For this review, take the finished solid that the model builds, in its own axes (mm). A direction names the side the tool comes from. Give positions to 0.01 mm unless a question says otherwise; leave off trailing zeros. Loops run counter-clockwise (first coordinate to the right, second up) from the corner with the lowest first, then second, coordinate; pieces in that order, holes last. Notation, with made-up numbers: (-35, 85.25) - (-5, 85.25) arc R16 ccw to (-5, 113.25) - close; hole circle Ø9 at (-12, 20). An arc over 180 degrees is marked (long way). Use CSV: the item, a comma, the result in double quotes. Start each with the question number.
1. Take a section at D-D on y = 1. Give the boundary of the cut face in (x, z), plus the area to 3 significant figures.
2. Take a section at A-A on x = 0. Give the boundary of the cut face in (y, z).
3. For faces 1 (the cylindrical face through (-26.2, 22.8, 10)), 2 (the cylindrical face through (28.549, 24.055, 1.452)), 3 (the flat face through (-11, 19.55, 0)), list the 3-axis set-ups (+Z, -Z, +X, -X, +Y, -Y) from which the entire face can be reached by the end or side of a thin tool; tool diameter is ignored.
4. Take a section at B-B on y = 9.25. Give the boundary of the cut face in (x, z).
5. For pin 1 (9.5 mm diameter, centred on y = 13, z = 0, fed in from -X); pin 2 (12 mm diameter, centred on y = 9, z = 2, fed in from +X); pin 3 (5 mm diameter, centred on y = 11, z = 2, fed in from +X); pin 4 (3 mm diameter, centred on x = 0, z = 0, fed in from -Y), all flat-tipped, find the tip position at first contact; note any pin that passes through.
6. Wall thickness on line 1 (Y direction, x = -28, z = 0); line 2 (Z direction, x = -21.5, y = 13.5); line 3 (X direction, y = 7.75, z = 1): over which ranges is each line inside the solid? List them lowest first.
7. Mouldability with a two-part tool opening along Z and no side actions: class faces 4 (the flat face through (-32, 2, -6)), 5 (the cylindrical face through (23.03, 5.19, 1.73)), 6 (the cylindrical face through (17, 27, 0)), 7 (the cylindrical face through (-1.2, 2.2, -7.9)) as pulls with the +Z half, pulls with the -Z half, needs draft (parallel to the pull), parting line crosses it, or undercut.
```python
from build123d import *

# Parameters (mm, degrees)
SKETCH1_R                       = 26
SKETCH1_R_2                     = 21.249999999999996
BOSS_EXTRUDE1_DEPTH             = 9
BOSS_EXTRUDE2_START             = 2
SKETCH2_R                       = 26.000000000000007
SKETCH2_R_2                     = 21.249999999999996
BOSS_EXTRUDE2_DEPTH             = 2
BOSS_EXTRUDE3_REACH             = 40.38
BOSS_EXTRUDE3_DIRECTION_2_DEPTH = 18
SKETCH4_R                       = 11.15
CUT_EXTRUDE1_DEPTH              = 7
CUT_EXTRUDE2_START              = -7
SKETCH5_R                       = 11.15
CUT_EXTRUDE2_DEPTH              = 7
FILLET2_R                       = 14
FILLET4_R                       = 1
SKETCH8_W                       = 43.8178046004133
SKETCH8_H                       = 27.999999999999993
BOSS_EXTRUDE4_DEPTH             = 11
SKETCH9_W                       = 43.8178046004133
SKETCH9_H                       = 11.999999999999998
CUT_EXTRUDE4_DEPTH              = 45.988887516807985
BOSS_EXTRUDE5_DEPTH             = 42.5
SKETCH6_R                       = 8
CUT_EXTRUDE3_DEPTH              = 65.6065012208524
BOSS_EXTRUDE6_START             = -4
BOSS_EXTRUDE6_DEPTH             = 42
SKETCH11_R                      = 2
CUT_EXTRUDE5_DEPTH              = 46.39823785126468
CUT_EXTRUDE6_DEPTH              = 51.36864114704705


with BuildPart() as part:
    # Sketch1 → Boss-Extrude1 (new body)
    with BuildSketch(Plane(origin=(0, 0, 0), x_dir=(1, 0, 0), z_dir=(0, 1, 0))):
        with Locations(Location((0, 0, 0), (0, 0, 270))):
            Circle(SKETCH1_R)
        with Locations(Location((0, 0, 0), (0, 0, 270))):
            Circle(SKETCH1_R_2, mode=Mode.SUBTRACT)
    extrude(amount=BOSS_EXTRUDE1_DEPTH)

    # Sketch2 → Boss-Extrude2 (add)
    with BuildSketch(Plane.XZ.offset(BOSS_EXTRUDE2_START)):
        with Locations(Location((0, 0, 0), (0, 0, 270))):
            Circle(SKETCH2_R)
        with Locations(Location((0, 0, 0), (0, 0, 270))):
            Circle(SKETCH2_R_2, mode=Mode.SUBTRACT)
    extrude(amount=-BOSS_EXTRUDE2_DEPTH)

    # Boss-Extrude3: up to this face of the body (flat: up to its plane)
    boss_extrude3_end = Plane(part.part.faces().sort_by_distance((0, -2, 25.264608948))[0])
    # Sketch3 → Boss-Extrude3 (add, up to the picked face)
    with BuildSketch(Plane(origin=(0, 9, 0), x_dir=(1, 0, 0), z_dir=(0, 1, 0)), mode=Mode.PRIVATE) as boss_extrude3_sk1:
        Polygon((21.249999999999996, 14.000000000000002), (32, 14.000000000000002), (32.00000000000001, -13.999999999999998), (21.250000000000004, -13.999999999999998), align=None)
    boss_extrude3_tool1 = split(extrude(boss_extrude3_sk1.sketch, amount=-BOSS_EXTRUDE3_REACH, mode=Mode.PRIVATE), bisect_by=boss_extrude3_end, keep=Keep.BOTH, mode=Mode.PRIVATE)
    # Sketch3 → Boss-Extrude3 (add, up to the picked face)
    with BuildSketch(Plane(origin=(0, 9, 0), x_dir=(1, 0, 0), z_dir=(0, 1, 0)), mode=Mode.PRIVATE) as boss_extrude3_sk2:
        Polygon((-32, 13.999999999999995), (-21.25, 13.999999999999995), (-21.250000000000004, -14.000000000000005), (-32, -14.000000000000004), align=None)
    boss_extrude3_tool2 = split(extrude(boss_extrude3_sk2.sketch, amount=-BOSS_EXTRUDE3_REACH, mode=Mode.PRIVATE), bisect_by=boss_extrude3_end, keep=Keep.BOTH, mode=Mode.PRIVATE)
    add(boss_extrude3_tool1.solids().sort_by(Axis((26.625, 9, 0), (0, -1, 0)))[0])
    add(boss_extrude3_tool2.solids().sort_by(Axis((-26.625, 9, 0), (0, -1, 0)))[0])

    # Sketch3 → Boss-Extrude3 direction 2 (add)
    with BuildSketch(Plane(origin=(0, 9, 0), x_dir=(1, 0, 0), z_dir=(0, 1, 0))):
        Polygon((21.249999999999996, 14.000000000000002), (32, 14.000000000000002), (32.00000000000001, -13.999999999999998), (21.250000000000004, -13.999999999999998), align=None)
        Polygon((-32, 13.999999999999995), (-21.25, 13.999999999999995), (-21.250000000000004, -14.000000000000005), (-32, -14.000000000000004), align=None)
    extrude(amount=BOSS_EXTRUDE3_DIRECTION_2_DEPTH)

    # Sketch4 → Cut-Extrude1 (cut)
    with BuildSketch(Plane(origin=(32.00000000000001, 0, -7.93e-15), x_dir=(-2.8e-16, 0, -1), z_dir=(1, 0, -2.8e-16))):
        with Locations((0, 12.999999999999998)):
            Circle(SKETCH4_R)
    extrude(amount=-CUT_EXTRUDE1_DEPTH, mode=Mode.SUBTRACT)

    # Sketch5 → Cut-Extrude2 (cut)
    with BuildSketch(Plane.ZY.offset(32).offset(CUT_EXTRUDE2_START)):
        with Locations(Location((-7.93e-15, 12.999999999999998, 0), (0, 0, 180))):
            Circle(SKETCH5_R)
    extrude(amount=CUT_EXTRUDE2_DEPTH, mode=Mode.SUBTRACT)

    # Fillet2
    fillet2_edges = [part.edges().sort_by_distance(p)[0] for p in [
        (-26.625, 27, 14.000000000000004),
        (-26.625, 27, -13.999999999999995),
        (26.625, 27, -14.000000000000002),
        (26.625000000000007, 27, 13.999999999999998),
    ]]
    fillet(fillet2_edges, radius=FILLET2_R - 0.0001)  # a hair under: the kernel refuses the full size

    # Fillet4
    fillet4_edges = [part.edges().sort_by_distance(p)[0] for p in [
        (-32, 3.5, 14.000000000000004),
        (-32, 3.5, -13.999999999999995),
        (-32, 22.89952422593355, -9.899524225933543),
        (-32, 22.899524225933547, 9.899524225933554),
        (32, 5.500050000000002, -14.000000000000004),
        (32.00000000000001, 5.500050000000002, 14),
        (32, 22.899524225933547, 9.89952422593355),
        (32, 22.89952422593355, -9.89952422593355),
    ]]
    fillet(fillet4_edges, radius=FILLET4_R)

    # Sketch8 → Boss-Extrude4 (add)
    with BuildSketch(Plane.XZ.offset(2)):
        Rectangle(SKETCH8_W, SKETCH8_H)
    extrude(amount=-BOSS_EXTRUDE4_DEPTH)

    # Sketch9 → Cut-Extrude4 (cut, through all)
    with BuildSketch(Plane(origin=(0, 9, 0), x_dir=(1, 0, 0), z_dir=(0, 1, 0))):
        Polygon((21.90890230020665, 14.000000000000002), (-21.908902300206655, 14.000000000000002), (-21.908902300206652, 25.999999999999996), (21.908902300206652, 25.999999999999996), align=None)
        with Locations((0, -20.000000000000004)):
            Rectangle(SKETCH9_W, SKETCH9_H)
    extrude(amount=-CUT_EXTRUDE4_DEPTH, mode=Mode.SUBTRACT)

    # Sketch12 → Boss-Extrude5 (add)
    with BuildSketch(Plane.ZY.offset(-21.25)):
        with BuildLine():
            Line((-13.999999999999996, 12.999999999999998), (-13.999999999999996, 9.000000000000002))
            Line((-13.999999999999996, 9.000000000000002), (14.00000000000001, 9))
            Line((14.00000000000001, 9), (14.000000000000004, 12.999999999999996))
            ThreePointArc((14.000000000000004, 12.999999999999996), (9.89949493661167, 22.89949493661166), (6.12e-15, 26.999999999999996))
            ThreePointArc((6.12e-15, 26.999999999999996), (-9.899494936611658, 22.89949493661166), (-13.999999999999996, 12.999999999999998))
        make_face()
    extrude(amount=BOSS_EXTRUDE5_DEPTH)

    # Sketch6 → Cut-Extrude3 (cut, through all)
    with BuildSketch(Plane(origin=(25.000000000000007, 0, -6.94e-15), x_dir=(-2.8e-16, 0, -1), z_dir=(1, 0, -2.8e-16))):
        with Locations((0, 12.999999999999998)):
            Circle(SKETCH6_R)
    extrude(amount=-CUT_EXTRUDE3_DEPTH, mode=Mode.SUBTRACT)

    # Sketch14 → Boss-Extrude6 (add)
    with BuildSketch(Plane(origin=(25.000000000000007, 0, -6.94e-15), x_dir=(-2.8e-16, 0, -1), z_dir=(1, 0, -2.8e-16)).offset(BOSS_EXTRUDE6_START)):
        with BuildLine():
            Line((-14.000000000000007, -2.0000000000000018), (-14.000000000000007, 12.999999999999996))
            ThreePointArc((-14.000000000000007, 12.999999999999996), (-9.899494936611672, 22.89949493661166), (-8.6e-15, 26.999999999999996))
            ThreePointArc((-8.6e-15, 26.999999999999996), (9.899494936611658, 22.89949493661166), (13.999999999999993, 12.999999999999996))
            Line((13.999999999999993, 12.999999999999996), (13.999999999999993, -2.0000000000000018))
            Line((13.999999999999993, -2.0000000000000018), (-14.000000000000007, -2.0000000000000018))
        make_face()
    extrude(amount=-BOSS_EXTRUDE6_DEPTH)

    # Sketch11 → Cut-Extrude5 (cut, through all)
    with BuildSketch(Plane.XZ.offset(2)):
        with Locations(Location((0, -9.5, 0), (0, 0, 270))):
            Circle(SKETCH11_R)
        with Locations(Location((0, 9.5, 0), (0, 0, 270))):
            Circle(SKETCH11_R)
        with Locations(Location((1.73e-15, -3.47e-15, 0), (0, 0, 270))):
            Circle(SKETCH11_R)
    extrude(amount=-CUT_EXTRUDE5_DEPTH, mode=Mode.SUBTRACT)

    # Sketch13 → Cut-Extrude6 (cut, through all)
    with BuildSketch(Plane(origin=(0, 0, -13.999999999999995), x_dir=(-1, 0, 0), z_dir=(0, 0, -1))):
        Polygon((15.547241809262866, 33.06287004539835), (15.54724180926287, 19.549999999999997), (0, 19.549999999999997), (-15.54724180926287, 19.549999999999994), (-15.54724180926287, 33.06287004539835), align=None)
        Polygon((6.549999999999999, 19.549999999999997), (0, 19.549999999999997), (-6.550000000000001, 19.549999999999997), (-6.55, 12.999999999999996), (6.550000000000001, 12.999999999999996), align=None)
        Polygon((6.550000000000001, 6.4499999999999975), (6.55, 12.999999999999996), (-6.549999999999997, 12.999999999999996), (-6.549999999999999, 6.4499999999999975), align=None)
    extrude(amount=-CUT_EXTRUDE6_DEPTH, mode=Mode.SUBTRACT)


solid = part.part
```
Check result:
1,outline,"(-32, -13) arc R1 ccw to (-31, -14) - (31, -14) arc R1 ccw to (32, -13) - (32, 13) arc R1 ccw to (31, 14) - (-31, 14) arc R1 ccw to (-32, 13) - close; hole circle Ø4 at (0, -9.5); hole circle Ø4 at (0, 0); hole circle Ø4 at (0, 9.5)"
1,area,"1,750 mm²"
2,outline,"(-2, -14) - (6.45, -14) - (6.45, -11.5) - (-2, -11.5) - close; (-2, -7.5) - (6.45, -7.5) - (6.45, -2) - (-2, -2) - close; (-2, 2) - (6.45, 2) - (6.45, 7.5) - (-2, 7.5) - close; (-2, 11.5) - (6.45, 11.5) - (6.45, 14) - (-2, 14) - close"
3,face 1,"+Z, +X, -X, +Y"
3,face 2,"+X"
3,face 3,"+Z, -Z, +Y"
4,outline,"(-32, -13) arc R1 ccw to (-31, -14) - (-6.55, -14) - (-6.55, 14) - (-31, 14) arc R1 ccw to (-32, 13) - (-32, 10.5) - (-25, 10.5) - (-25, 7.07) - (-21, 7.07) - (-21, -7.07) - (-25, -7.07) - (-25, -10.5) - (-32, -10.5) - close; (6.55, -14) - (31, -14) arc R1 ccw to (32, -13) - (32, -10.5) - (25, -10.5) - (25, -7.07) - (21, -7.07) - (21, 7.07) - (25, 7.07) - (25, 10.5) - (32, 10.5) - (32, 13) arc R1 ccw to (31, 14) - (6.55, 14) - close"
5,pin 1,"stops at x = -21"
5,pin 2,"stops at x = 25"
5,pin 3,"stops at x = 21"
5,pin 4,"passes through"
6,line 1,"y = -2 to 1.85, 24.15 to 27"
6,line 2,"z = -13.99 to -7.98, 7.98 to 13.99"
6,line 3,"x = -21 to -6.55, 6.55 to 21"
7,face 4,"needs draft"
7,face 5,"undercut"
7,face 6,"parting line crosses it"
7,face 7,"undercut"
